Work out the finished part from the listing and answer in its coordinate system (mm). Give positions to 0.01 mm unless a question says otherwise; leave off trailing zeros. Write each loop counter-clockwise with the first axis right and the second up, starting at its lowest first coordinate (ties: lowest second). Pieces come first, ordered by that corner, then holes. Notation, with made-up numbers: (66, 41.25) -> (111, 41.25) arc R15 cw to (111, 62.25) -> close; hole circle Ø8 at (89.5, 70.5). An arc over 180 degrees is marked (long way). Write item = value, one per line. Start each with the question number.
from build123d import *

# Parameters (mm, degrees)
F2_R = 5.99999


# Not quite as in the source:
# - a fillet or chamfer is up to 0.001 mm smaller than in the source, because OpenCascade refuses the exact size


with BuildPart() as f1:
    # F0 (on Front) → F1 (revolve)
    with BuildSketch(Plane.XZ):
        Polygon((-109.55, 0), (0, 0), (0, 37), (-87.33, 37), (-87.33, 43), (-88.33, 43), (-109.55, 27.0095830568), align=None)
    revolve(axis=Axis((0, 0, 18.5), (0, 0, 1)))

    # F2 (radius 6 in the source; OpenCascade refuses exactly that, so slightly less here)
    f2_edges = [f1.edges().sort_by_distance(p)[0] for p in [
        (87.33, 0, 37),
    ]]
    fillet(f2_edges, radius=F2_R)


solid = f1.part
(1) Find the intervals of material crossed by line 1 along Z through (x, y) = (61, -44.5); line 2 along X through (y, z) = (21, 39); line 3 along Y through (x, z) = (26, 39), in increasing order.
(2) Determine the mould class of faces 1 (the conical face through (-85.52, -26.93, 42)), 2 (the flat face through (2, -2, 0)), 3 (the flat face through (-1, -1, 37)) for opening direction X: pulls with the +X half, pulls with the -X half, needs draft (parallel to the pull), parting line crosses it, or undercut.
(3) A cutting plane is placed at C-C, the plane z = 3. Write down the section's boundary in (x, y).
(4) A cutting plane is placed at D-D, the plane z = 31.5. Write down the section's boundary in (x, y), then the cut area to 3 significant figures.
(5) Each of these flat-tipped pins is pushed along its axis until it touches: pin 1 (2 mm diameter, centred on x = -47.5, z = 16, fed in from -Y); pin 2 (8 mm diameter, centred on x = -34.5, z = 20, fed in from -Y); pin 3 (10 mm diameter, centred on y = -19, z = 18.5, fed in from +X). Where does it stop, or does it pass through?
Results list:
q1.line_1 = 0 to 37
q1.line_2 = -91.25 to -83.19, 83.19 to 91.25
q1.line_3 = -89.96 to -81.77, 81.77 to 89.96
q2.face_1 = parting line crosses it
q2.face_2 = needs draft
q2.face_3 = undercut
q3.outline = circle Ø219.1 at (0, 0)
q4.outline = circle Ø207.18 at (0, 0)
q4.area = 33,700 mm²
q5.pin_1 = -99.19
q5.pin_2 = -105.22
q5.pin_3 = 108.65
